Read the model definition and answer for the solid it produces. Units are mm, in the model's axes. Coordinates: 2 decimals unless noted, no trailing zeros. Write each loop counter-clockwise with the first axis right and the second up, starting at its lowest first coordinate (ties: lowest second). Pieces come first, ordered by that corner, then holes. Notation, with made-up numbers: (-19.5, 40.25) -> (3.5, 40.25) arc R23 ccw to (3.5, 59.25) -> close; hole circle Ø7 at (53, -22). An arc over 180 degrees is marked (long way). Write item = value, one per line. Start each with the question number.
1) Find the intervals of material crossed by line 1 along Z through (x, y) = (48.5, -0.7); line 2 along X through (y, z) = (-1, -77); line 3 along X through (y, z) = (-0.3, -44), in increasing order. Write a range as from..to.
2) Section B-B (z = -57) is taken. Determine the outline of the cut face in (x, y).
3) Flat-ended cylindrical pins translate along their axes: pin 1 Ø3 at (x, z) = (7, -5.5) entering from +Y; pin 2 Ø3 at (x, z) = (-8.595, -38.5) entering from -Y. Find the tip coordinate at first contact, or state that the pin passes through.
4) For a pull along X with two mould halves and no side action, classify faces 1 (the face through (47.696, -0.74, -55.463)), 2 (the face through (60, -1.5, -38)) as released by +X, released by -X, zero draft, split by the parting line, or undercut.
5) Section C-C (y = -1.25) is taken. Count the separate pieces of the cut face and the enclosed holes in it, plus the area to 3 significant figures.
6) Section A-A (z = -38.5) is taken. Determine the outline of the cut face in (x, y) (3 decimals).
Autodesk Inventor part; units mm, degrees
ref_plane "YZ Plane" through (0, 0, 0) normal (1, 0, 0) x (0, 1, 0)
ref_plane "XZ Plane" through (0, 0, 0) normal (0, 1, 0) x (-1, 0, 0)
ref_plane "XY Plane" through (0, 0, 0) normal (0, 0, 1) x (1, 0, 0)
sketch "Sketch1" plane through (0, 0, 0) normal (0, 1, 0) x (-1, 0, 0)
  line L0 (-0.4496, -47) -> (-0.4496, 0)
  line L1 (-117.7289, 0) -> (-117.7289, -47)
  circle A0 centre (-97.2793, 2) radius 1.55
  circle A1 centre (-97.2793, -43) radius 1.55
  circle A2 centre (-20.8993, 2) radius 1.55
  circle A3 centre (-20.8993, -43) radius 1.55
  circle A4 centre (-70.6843, -57) radius 1.55
  circle A5 centre (-47.4943, -57) radius 1.55
  circle A6 centre (-47.4943, -77) radius 1.55
  circle A7 centre (-70.6843, -77) radius 1.55
  circle A8 centre (-97.0893, -77.595) radius 1.55
  circle A9 centre (-21.5893, -77.595) radius 1.55
  circle A10 centre (-126.7736, -8.5) radius 1.55
  circle A11 centre (8.595, -8.5) radius 1.55
  circle A12 centre (-126.7736, -38.5) radius 1.55
  circle A13 centre (8.595, -38.5) radius 1.55
  arc A14 (17.19, -47) -> (18.19, -46) centre (17.19, -46) ccw
  line L2 (18.19, -1) -> (18.19, -46)
  arc A15 (-1.5893, -87) -> (-0.5893, -86) centre (-1.5893, -86) ccw
  line L3 (-0.5893, -48.5) -> (-0.5893, -86)
  arc A16 (-117.5893, -86) -> (-116.5893, -87) centre (-116.5893, -86) ccw
  line L4 (-117.5893, -86) -> (-117.5893, -48.5)
  arc A17 (-136.3686, -46) -> (-135.3686, -47) centre (-135.3686, -46) ccw
  arc A18 (-135.3686, 0) -> (-136.3686, -1) centre (-135.3686, -1) ccw
  line L5 (-135.3686, 0) -> (-116.5293, 0)
  arc A19 (-116.5893, 10) -> (-117.5893, 9) centre (-116.5893, 9) ccw
  line L6 (-116.5893, 10) -> (-1.5893, 10)
  arc A20 (-0.5893, 9) -> (-1.5893, 10) centre (-1.5893, 9) ccw
  arc A21 (18.19, -1) -> (17.19, 0) centre (17.19, -1) ccw
  line L7 (-136.3686, -46) -> (-136.3686, -1)
  line L8 (17.19, -47) -> (-1.6493, -47)
  line L9 (-1.6493, 0) -> (17.19, 0)
  line L10 (-1.6493, 0) -> (-1.6493, 1.5)
  line L11 (-1.6493, 1.5) -> (-0.5893, 1.5)
  line L12 (-0.5893, 9) -> (-0.5893, 1.5)
  line L13 (-117.5893, 1.5) -> (-117.5893, 9)
  line L14 (-117.5893, 1.5) -> (-116.5293, 1.5)
  line L15 (-116.5293, 1.5) -> (-116.5293, 0)
  line L16 (-116.5293, -47) -> (-135.3686, -47)
  line L17 (-116.5293, -47) -> (-116.5293, -48.5)
  line L18 (-116.5293, -48.5) -> (-117.5893, -48.5)
  line L19 (-1.5893, -87) -> (-116.5893, -87)
  line L20 (-0.5893, -48.5) -> (-1.6493, -48.5)
  line L21 (-1.6493, -48.5) -> (-1.6493, -47)
  line L22 (-118.1786, -47) -> (-118.1786, 0)
  line L23 (-117.2793, 0) -> (-117.2793, -47)
  line L24 (-0.8993, -47) -> (-0.8993, 0)
  line L25 (0, 0) -> (0, -47)
extrude "Extrusion1" add sketch "Sketch1" against normal blind 1.5
properties part number "body_front_frame"
Answer key:
q1.line_1 = -87..-78.18, -75.82..-58.18, -55.82..10
q1.line_2 = 0.59..20.16, 23.02..45.94, 49.04..69.13, 72.23..95.66, 98.52..117.59
q1.line_3 = -18.19..19.72, 22.08..96.1, 98.46..136.37
q2.outline = (0.59, -1.5) -> (45.94, -1.5) -> (45.94, 0) -> (0.59, 0) -> close; (49.04, -1.5) -> (69.13, -1.5) -> (69.13, 0) -> (49.04, 0) -> close; (72.23, -1.5) -> (117.59, -1.5) -> (117.59, 0) -> (72.23, 0) -> close
q3.pin_1 = 0
q3.pin_2 = through
q4.face_1 = undercut
q4.face_2 = zero draft
q5.separate_pieces = 1
q5.enclosed_holes = 14
q5.area = 13,000 mm^2
q6.outline = (-18.19, -1.5) -> (-10.145, -1.5) -> (-10.145, 0) -> (-18.19, 0) -> close; (-7.045, -1.5) -> (125.224, -1.5) -> (125.224, 0) -> (-7.045, 0) -> close; (128.324, -1.5) -> (136.369, -1.5) -> (136.369, 0) -> (128.324, 0) -> close
